Read the model definition and answer for the solid it produces. Units are mm, in the model's axes. A direction names the side the tool comes from. Give positions to 0.01 mm unless a question says otherwise; leave off trailing zeros. Write each loop counter-clockwise with the first axis right and the second up, starting at its lowest first coordinate (ties: lowest second). Pieces come first, ordered by that corner, then holes. Notation, with made-up numbers: (-6, 75.5) - (49, 75.5) arc R13 cw to (49, 88.5) - close; hole circle Ø1 at (68.25, 16). An arc over 180 degrees is marked (long way). Answer as CSV lines item,"result".
```python
from build123d import *

# Parameters (mm, degrees)
BOSS_EXTRUDE1_DEPTH = 508
FILLET1_R           = 1.651


with BuildPart() as part:
    # Sketch1 → Boss-Extrude1 (new body)
    with BuildSketch(Plane.XY):
        with BuildLine():
            Line((0, 0), (-1.969087929, 0))
            ThreePointArc((-1.969087929, 0), (-4.754845979, 2.586764816), (-2.38125, 5.55625))
            Line((-2.38125, 5.55625), (-2.38125, 10.590485541))
            ThreePointArc((-2.38125, 10.590485541), (-3.532318917, 14.479050507), (-6.614583333, 17.11449036))
            ThreePointArc((-6.614583333, 17.11449036), (-12.779112166, 22.385370067), (-15.08125, 30.1625))
            Line((-15.08125, 30.1625), (-17.4625, 30.1625))
            ThreePointArc((-17.4625, 30.1625), (-19.200240239, 35.281057809), (-23.8125, 38.1))
            Line((-23.8125, 38.1), (-23.8125, 50.8))
            Line((-23.8125, 50.8), (0, 50.8))
            Line((0, 50.8), (0, 49.149))
            Line((0, 49.149), (-22.1615, 49.149))
            Line((-22.1615, 49.149), (-22.1615, 39.348165423))
            ThreePointArc((-22.1615, 39.348165423), (-18.011172085, 36.435510418), (-15.926513678, 31.8135))
            Line((-15.926513678, 31.8135), (-13.321931482, 31.8135))
            ThreePointArc((-13.321931482, 31.8135), (-11.821707612, 23.992793107), (-5.941953704, 18.622260363))
            ThreePointArc((-5.941953704, 18.622260363), (-2.147343733, 15.377741077), (-0.73025, 10.590485541))
            Line((-0.73025, 10.590485541), (-0.73025, 5.174662071))
            ThreePointArc((-0.73025, 5.174662071), (-1.093097229, 4.29867137), (-1.969087929, 3.935824141))
            ThreePointArc((-1.969087929, 3.935824141), (-3.1115, 2.793412071), (-1.969087929, 1.651))
            Line((-1.969087929, 1.651), (0, 1.651))
            Line((0, 1.651), (0, 0))
        make_face()
    extrude(amount=-BOSS_EXTRUDE1_DEPTH)

    # Fillet1
    fillet1_edges = [part.edges().sort_by_distance(p)[0] for p in [
        (-17.4625, 30.1625, -254),
        (-23.8125, 38.1, -254),
        (-23.8125, 50.8, -254),
        (-13.321931482, 31.8135, -254),
    ]]
    fillet(fillet1_edges, radius=FILLET1_R)


solid = part.part
```
(1) A cutting plane is placed at A-A (z = -101.5). Write down the section's boundary in (x, y) (1 decimal), and give its area (3 significant figures).
Worked out:
outline,"(-23.8, 39.3) arc R1.7 ccw to (-22.7, 37.8) arc R7.9 cw to (-17.6, 31.6) arc R1.7 ccw to (-15.9, 30.2) - (-15.1, 30.2) arc R14.3 ccw to (-6.6, 17.1) arc R7.1 cw to (-2.4, 10.6) - (-2.4, 5.6) arc R2.8 ccw to (-2, 0) - (0, 0) - (0, 1.7) - (-2, 1.7) arc R1.1 cw to (-2, 3.9) arc R1.2 ccw to (-0.7, 5.2) - (-0.7, 10.6) arc R8.8 ccw to (-5.9, 18.6) arc R12.6 cw to (-13.4, 30.2) arc R1.7 ccw to (-15.1, 31.8) - (-15.9, 31.8) arc R9.6 ccw to (-22.2, 39.3) - (-22.2, 49.1) - (0, 49.1) - (0, 50.8) - (-22.2, 50.8) arc R1.7 ccw to (-23.8, 49.1) - close"
area,"142 mm^2"
(2) For faces 4 (the flat face through (-14, 31, 0)), 5 (the cylindrical face through (-11.45, 23.37, -250.44)), determine the directions among +Z, -Z, +X, -X, +Y, -Y from which every point of the face is accessible in a straight line to the end or side of a thin tool.
Worked out:
face 4,"+Z, +X, -X, +Y, -Y"
face 5,"+Z, -Z, +X"
(3) Find the intervals of material crossed by L1, parallel to Y at x = -22.5, z = -78; L2, parallel to X at y = 7, z = -275; L3, parallel to Y at x = -18.5, z = -205.5, in increasing order.
Worked out:
L1,"y = 37.71 to 50.76"
L2,"x = -2.38 to -0.73"
L3,"y = 34.25 to 36.98, 49.15 to 50.8"
(4) A cutting plane is placed at B-B (y = 44). Write down the section's boundary in (x, z).
Worked out:
outline,"(-23.81, -508) - (-22.16, -508) - (-22.16, 0) - (-23.81, 0) - close"
(5) The mould has two halves that part along Y. Classify faces 1 (the flat face through (-23.812, 44, -250)), 2 (the cylindrical face through (-12.716, 22.289, -250.444)), 3 (the flat face through (-11, 49.149, -250)): +Y half, -Y half, draft (parallel to the pull), parting line (faces both ways), or undercut.
Worked out:
face 1,"draft"
face 2,"-Y half"
face 3,"undercut"
(6) Each of these flat-tipped pins is pushed along its axis until it touches: P1, Ø1.5, axis at y = 36.5, z = -329.5, coming from the -X side; P2, Ø1.5, axis at y = 8.5, z = -237.5, coming from the -X side; P3, Ø1.5, axis at x = -19, y = 33, coming from the -Z side; P4, Ø6, axis at y = 38, z = -371.5, coming from the +X side. Where does it stop, or does it pass through?
Worked out:
P1,"stops at x = -21.52"
P2,"stops at x = -2.38"
P3,"passes through"
P4,"stops at x = -17.03"
(7) A cutting plane is placed at C-C (y = 23). Write down the section's boundary in (x, z).
Worked out:
outline,"(-13.16, -508) - (-11.2, -508) - (-11.2, 0) - (-13.16, 0) - close"
